```python
from build123d import *

# Parameters (mm, degrees)
SKETCH1_R           = 1.5
SKETCH1_R_2         = 1.56
BOSS_EXTRUDE1_DEPTH = 3


with BuildPart() as part:
    # Sketch1 → Boss-Extrude1 (new body)
    with BuildSketch(Plane.XY):
        with BuildLine():
            Line((-75, 50), (75, 50))
            ThreePointArc((75, 50), (82.071067812, 47.071067812), (85, 40))
            Line((85, 40), (85, -40))
            ThreePointArc((85, -40), (82.071067812, -47.071067812), (75, -50))
            Line((75, -50), (-75, -50))
            ThreePointArc((-75, -50), (-82.071067812, -47.071067812), (-85, -40))
            Line((-85, -40), (-85, 40))
            ThreePointArc((-85, 40), (-82.071067812, 47.071067812), (-75, 50))
        make_face()
        with Locations((-75, 40)):
            Circle(SKETCH1_R, mode=Mode.SUBTRACT)
        with Locations((75, 40)):
            Circle(SKETCH1_R, mode=Mode.SUBTRACT)
        with Locations((75, -40)):
            Circle(SKETCH1_R, mode=Mode.SUBTRACT)
        with Locations((-75, -40)):
            Circle(SKETCH1_R, mode=Mode.SUBTRACT)
        with Locations((0, 19)):
            Circle(SKETCH1_R_2, mode=Mode.SUBTRACT)
        with Locations((0, -19)):
            Circle(SKETCH1_R_2, mode=Mode.SUBTRACT)
        with BuildLine():
            Line((-25, 46.257829906), (25, 46.257829906))
            ThreePointArc((25, 46.257829906), (30, 41.257829906), (25, 36.257829906))
            Line((25, 36.257829906), (-25, 36.257829906))
            ThreePointArc((-25, 36.257829906), (-30, 41.257829906), (-25, 46.257829906))
        make_face(mode=Mode.SUBTRACT)
        with BuildLine():
            Line((-25, -46.257829906), (25, -46.257829906))
            ThreePointArc((25, -46.257829906), (30, -41.257829906), (25, -36.257829906))
            Line((25, -36.257829906), (-25, -36.257829906))
            ThreePointArc((-25, -36.257829906), (-30, -41.257829906), (-25, -46.257829906))
        make_face(mode=Mode.SUBTRACT)
    extrude(amount=BOSS_EXTRUDE1_DEPTH)


solid = part.part
```
Read the model definition and answer for the solid it produces. Units are mm, in the model's axes. A direction names the side the tool comes from. Coordinates: 2 decimals unless noted, no trailing zeros. Answer as a JSON object with one key per item and string values. Group by question number.
1. A cutting plane is placed at A-A (z = 2.05). Give the number of separate pieces and of enclosed holes in the cut face, plus the area to 3 significant figures.
2. Which of the six approach directions +Z, -Z, +X, -X, +Y, -Y give full straight-line access (tool end or side, diameter ignored) to faces 4 (the cylindrical face through (82.15, -46.99, 1.48)), 5 (the flat face through (0, 46.258, 1))?
3. Consider L1, parallel to Y at x = 0, z = 1.55; L2, parallel to Y at x = -7.5, z = 1.95; L3, parallel to Y at x = -75, z = 1.9. Determine where each line is inside the solid, lowest interval first. Write a range as [from, to].
4. The mould has two halves that part along Y. Classify faces 1 (the flat face through (1, -50, 1)), 2 (the cylindrical face through (-1.238, -19.949, 1.479)), 3 (the flat face through (1, 1, 3)): +Y half, -Y half, draft (parallel to the pull), parting line (faces both ways), or undercut.
Worked out:
{
 "1": {"separate pieces": "1", "enclosed holes": "8", "area": "15,700 mm²"},
 "2": {"face 4": "+Z, -Z, +X, -Y", "face 5": "+Z, -Z"},
 "3": {"L1": "y = [-50, -46.26], [-36.26, -20.56], [-17.44, 17.44], [20.56, 36.26], [46.26, 50]", "L2": "y = [-50, -46.26], [-36.26, 36.26], [46.26, 50]", "L3": "y = [-50, -41.5], [-38.5, 38.5], [41.5, 50]"},
 "4": {"face 1": "-Y half", "face 2": "undercut", "face 3": "draft"}
}
